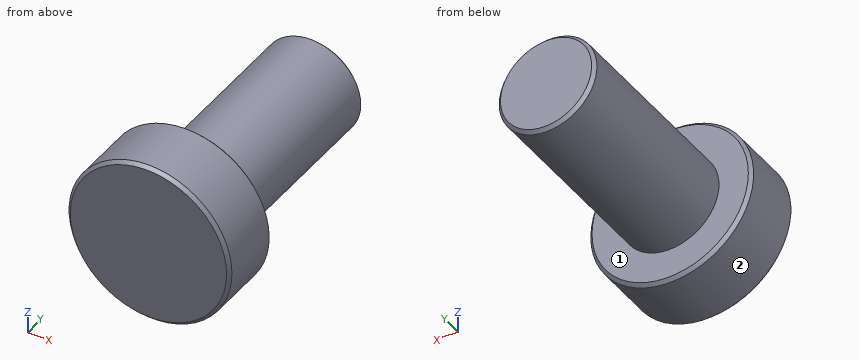
from build123d import *

# Parameters (mm, degrees)
SKETCH_1_R      = 5
EXTRUDE_1_DEPTH = 4
SKETCH_2_R      = 3
EXTRUDE_2_DEPTH = 12
CHAMFER_1_SIZE  = 0.2


with BuildPart() as part:
    # Эскиз1 → Бобышка-Вытянуть1 (new body)
    with BuildSketch(Plane(origin=(0, 0, 0), x_dir=(1, 0, 0), z_dir=(0, 1, 0))):
        Circle(SKETCH_1_R)
    extrude(amount=EXTRUDE_1_DEPTH)

    # Эскиз2 → Бобышка-Вытянуть2 (add)
    with BuildSketch(Plane(origin=(0, 4, 0), x_dir=(1, 0, 0), z_dir=(0, 1, 0))):
        Circle(SKETCH_2_R)
    extrude(amount=EXTRUDE_2_DEPTH)

    # Фаска1
    chamfer_1_edges = [part.edges().sort_by_distance(p)[0] for p in [
        (-5, 0, 0),
        (-5, 4, 0),
        (-3, 16, 0),
    ]]
    chamfer(chamfer_1_edges, length=CHAMFER_1_SIZE)


solid = part.part
Input: part model. Units: mm. Frame: model coordinates. Face numbers are marked on the shaded views. A direction names the side the tool comes from. Give positions to 0.01 mm unless a question says otherwise; leave off trailing zeros. Loops run counter-clockwise (first coordinate to the right, second up) from the corner with the lowest first, then second, coordinate; pieces in that order, holes last. Notation, with made-up numbers: (42.5, 8.25) -> (52.5, 8.25) arc R12 cw to (52.5, 30.25) -> close; hole circle Ø7 at (-20.5, 47.25). An arc over 180 degrees is marked (long way). Answer as a JSON object with one key per item and string values. Group by question number.
Item 1: Cut plane D-D, the plane y = 14.5. Return the cut outline in (x, z), and give its area (3 significant figures).
Item 2: Cut plane B-B, the plane x = 0. Return the cut outline in (y, z).
Item 3: Reachability of the marked faces 1 and 2 from +Z, -Z, +X, -X, +Y, -Y: full face, straight path, thin tool, end or side. Return the list, or none.
Item 4: Line query: probe 1 along Y at (x, z) = (-2.5, -2); probe 2 along X at (y, z) = (14.5, -2.25); probe 3 along X at (y, z) = (10.75, 1). Output: solid intervals per line, ascending.
Item 5: Pin query (flat end, axial travel): P1, Ø1, axis at y = 10, z = 0, coming from the +X side; P2, Ø1.5, axis at x = -2.5, y = 2.5, coming from the +Z side; P3, Ø5, axis at y = 12, z = 2, coming from the -X side. Return the tip coordinate at first contact, or that it passes through.
Item 6: Cut plane C-C, the plane y = 1.75. Return the cut outline in (x, z), and give its area (3 significant figures).
Item 7: Cut plane A-A, the plane z = 0. Return the cut outline in (x, y), and give its area (3 significant figures).
Checks:
{
 "1": {"outline": "circle Ø6 at (0, 0)", "area": "28.3 mm²"},
 "2": {"outline": "(0, -4.8) -> (0.2, -5) -> (3.8, -5) -> (4, -4.8) -> (4, -3) -> (15.8, -3) -> (16, -2.8) -> (16, 2.8) -> (15.8, 3) -> (4, 3) -> (4, 4.8) -> (3.8, 5) -> (0.2, 5) -> (0, 4.8) -> close"},
 "3": {"face 1": "+Y", "face 2": "+Y, -Y"},
 "4": {"probe 1": "y = 0 to 4", "probe 2": "x = -1.98 to 1.98", "probe 3": "x = -2.83 to 2.83"},
 "5": {"P1": "stops at x = 3", "P2": "stops at z = 4.68", "P3": "stops at x = -3"},
 "6": {"outline": "circle Ø10 at (0, 0)", "area": "78.5 mm²"},
 "7": {"outline": "(-5, 0.2) -> (-4.8, 0) -> (4.8, 0) -> (5, 0.2) -> (5, 3.8) -> (4.8, 4) -> (3, 4) -> (3, 15.8) -> (2.8, 16) -> (-2.8, 16) -> (-3, 15.8) -> (-3, 4) -> (-4.8, 4) -> (-5, 3.8) -> close", "area": "112 mm²"}
}
